from build123d import *

# Parameters (mm, degrees)
SM_BASE_FLANGE_1_DEPTH = 30
CUT_EXTRUDE_1_DEPTH    = 10
CUT_EXTRUDE_2_DEPTH    = 10
FILLET_1_R             = 2


# Sheet-metal steps are written as plain solids
with BuildPart() as part:
    # Sketch 1 → 基体-法兰1 (new body)
    with BuildSketch(Plane.XY):
        with BuildLine():
            Line((0, 19), (0, 4))
            ThreePointArc((0, 4), (1.171572875, 1.171572875), (4, 0))
            Line((4, 0), (32, 0))
            Line((32, 0), (32, 2))
            Line((32, 2), (4, 2))
            ThreePointArc((4, 2), (2.585786438, 2.585786438), (2, 4))
            Line((2, 4), (2, 19))
            Line((2, 19), (0, 19))
        make_face()
    extrude(amount=SM_BASE_FLANGE_1_DEPTH)

    # 草图6 → 切除-拉伸1 (cut)
    with BuildSketch(Plane.ZY):
        with BuildLine():
            Line((23.45, 8), (23.45, 12))
            ThreePointArc((23.45, 12), (25, 13.55), (26.55, 12))
            Line((26.55, 12), (26.55, 8))
            ThreePointArc((26.55, 8), (25, 6.45), (23.45, 8))
        make_face()
        with BuildLine():
            Line((13.45, 8), (13.45, 12))
            ThreePointArc((13.45, 12), (15, 13.55), (16.55, 12))
            Line((16.55, 12), (16.55, 8))
            ThreePointArc((16.55, 8), (15, 6.45), (13.45, 8))
        make_face()
        with BuildLine():
            Line((3.45, 8), (3.45, 12))
            ThreePointArc((3.45, 12), (5, 13.55), (6.55, 12))
            Line((6.55, 12), (6.55, 8))
            ThreePointArc((6.55, 8), (5, 6.45), (3.45, 8))
        make_face()
    extrude(amount=-CUT_EXTRUDE_1_DEPTH, mode=Mode.SUBTRACT)

    # 草图10 → 切除-拉伸2 (cut)
    with BuildSketch(Plane(origin=(0, 2, 0), x_dir=(1, 0, 0), z_dir=(0, 1, 0))):
        with BuildLine():
            Line((24, -27.05), (18, -27.05))
            ThreePointArc((18, -27.05), (15.95, -25), (18, -22.95))
            Line((18, -22.95), (24, -22.95))
            ThreePointArc((24, -22.95), (26.05, -25), (24, -27.05))
        make_face()
        with BuildLine():
            Line((24, -17.05), (18, -17.05))
            ThreePointArc((18, -17.05), (15.95, -15), (18, -12.95))
            Line((18, -12.95), (24, -12.95))
            ThreePointArc((24, -12.95), (26.05, -15), (24, -17.05))
        make_face()
        with BuildLine():
            Line((24, -7.05), (18, -7.05))
            ThreePointArc((18, -7.05), (15.95, -5), (18, -2.95))
            Line((18, -2.95), (24, -2.95))
            ThreePointArc((24, -2.95), (26.05, -5), (24, -7.05))
        make_face()
    extrude(amount=-CUT_EXTRUDE_2_DEPTH, mode=Mode.SUBTRACT)

    # 圆角1
    fillet_1_edges = [part.edges().sort_by_distance(p)[0] for p in [
        (1, 19, 30),
        (1, 19, 0),
        (32, 1, 30),
        (32, 1, 0),
    ]]
    fillet(fillet_1_edges, radius=FILLET_1_R)


solid = part.part
Input: part model. Units: mm. Frame: model coordinates. A direction names the side the tool comes from. Round coordinates to 2 decimals unless told otherwise and drop trailing zeros. Order: outer loops, then holes, each group sorted by start corner. A loop starts at its lowest first (then second) coordinate and runs counter-clockwise, first axis right, second up. Notation, with made-up numbers: (83.25, 0.25) - (101.25, 0.25) arc R35 cw to (101.25, 32.25) - close; hole circle Ø9 at (63, 9.25). An arc over 180 degrees is marked (long way). Answer as a JSON object with one key per item and string values. Group by question number.
(1) Cut plane A-A (z = 15). Return loops of the section in (x, y).
(2) Cut plane B-B (y = 11). Return loops of the section in (x, z), then the cut area to 3 significant figures.
(3) Cut plane D-D (z = 9.25). Return loops of the section in (x, y), then the cut area to 3 significant figures.
(4) Reachability of faces 4 (the face through (2, 15, 15)), 5 (the face through (21, 1, 27.05)), 6 (the face through (0.99, 13.55, 24.97)), 7 (the face through (9.4, 1.6, 0)) from +Z, -Z, +X, -X, +Y, -Y: full face, straight path, thin tool, end or side. Return the list, or none.
(5) Draft query along Y for faces 1 (the face through (0, 15, 15)), 2 (the face through (0.99, 13.55, 4.97)), 3 (the face through (0.99, 18.43, 0.6)). Return one class per face: released by +Y, released by -Y, zero draft, split by the parting line, or undercut.
(6) Cut plane C-C (x = 22.5). Return loops of the section in (y, z), then the cut area to 3 significant figures.
(7) Material intervals for probe 1 along X at (y, z) = (17.25, 28); probe 2 along X at (y, z) = (2.5, 6.5), sorted ascending. Write a range as from..to.
(8) Pin query (flat end, axial travel): P1, Ø8, axis at x = 26, z = 18, coming from the +Y side; P2, Ø6, axis at x = 4, y = 5, coming from the -Z side; P3, Ø6, axis at y = 11, z = 18.5, coming from the +X side; P4, Ø3, axis at x = 21, z = 25.5, coming from the +Y side. Return the tip coordinate at first contact, or that it passes through.
Here are the results:
{
 "1": {"outline": "(0, 4) arc R4 ccw to (4, 0) - (15.95, 0) - (15.95, 2) - (4, 2) arc R2 cw to (2, 4) - (2, 6.45) - (0, 6.45) - close; (0, 13.55) - (2, 13.55) - (2, 19) - (0, 19) - close; (26.05, 0) - (32, 0) - (32, 2) - (26.05, 2) - close"},
 "2": {"outline": "(0, 0) - (2, 0) - (2, 3.45) - (0, 3.45) - close; (0, 6.55) - (2, 6.55) - (2, 13.45) - (0, 13.45) - close; (0, 16.55) - (2, 16.55) - (2, 23.45) - (0, 23.45) - close; (0, 26.55) - (2, 26.55) - (2, 30) - (0, 30) - close", "area": "41.4 mm^2"},
 "3": {"outline": "(0, 4) arc R4 ccw to (4, 0) - (32, 0) - (32, 2) - (4, 2) arc R2 cw to (2, 4) - (2, 19) - (0, 19) - close", "area": "95.4 mm^2"},
 "4": {"face 4": "+Z, -Z, +X, +Y", "face 5": "+Y, -Y", "face 6": "+X, -X", "face 7": "-Z, +X, -X, +Y, -Y"},
 "5": {"face 1": "zero draft", "face 2": "undercut", "face 3": "released by +Y"},
 "6": {"outline": "(0, 0) - (2, 0) - (2, 2.95) - (0, 2.95) - close; (0, 7.05) - (2, 7.05) - (2, 12.95) - (0, 12.95) - close; (0, 17.05) - (2, 17.05) - (2, 22.95) - (0, 22.95) - close; (0, 27.05) - (2, 27.05) - (2, 30) - (0, 30) - close", "area": "35.4 mm^2"},
 "7": {"probe 1": "x = 0..2", "probe 2": "x = 0.29..2.68"},
 "8": {"P1": "stops at y = 2", "P2": "stops at z = 0", "P3": "stops at x = 2", "P4": "passes through"}
}
